from build123d import *

# Parameters (mm, degrees)
MODEL_R         = 0.65
MODEL_R_2       = 3.4746057
EXTRUDE_1_DEPTH = 0.5
EXTRUDE2_START  = -0.1
SKETCH2_R       = 0.65
SKETCH2_W       = 3.5
SKETCH2_H       = 2
EXTRUDE2_DEPTH  = 0.1
EXTRUDE1_START  = -0.5
EXTRUDE1_DEPTH  = 0.9


# Read off the part's stored shape, not the designer's step: Extrude1
with BuildPart() as part:
    # Model → Бобышка-Вытянуть1 (new, symmetric)
    with BuildSketch(Plane.XY):
        with BuildLine():
            Line((1024.38859, -762.8000398), (1024.38859, -762.0000398))
            Line((1024.38859, -762.0000398), (1012.53859, -762.0000398))
            Line((1012.53859, -762.0000398), (1012.53859, -773.0000398))
            Line((1012.53859, -773.0000398), (1024.38859, -773.0000398))
            Line((1024.38859, -773.0000398), (1024.38859, -772.2000398))
            ThreePointArc((1024.38859, -772.2000398), (1025.03859, -771.5500398), (1025.68859, -772.2000398))
            Line((1025.68859, -772.2000398), (1025.68859, -773.0000398))
            Line((1025.68859, -773.0000398), (1035.03859, -773.0000398))
            Line((1035.03859, -773.0000398), (1035.03859, -762.0000398))
            Line((1035.03859, -762.0000398), (1025.68859, -762.0000398))
            Line((1025.68859, -762.0000398), (1025.68859, -762.8000398))
            ThreePointArc((1025.68859, -762.8000398), (1025.03859, -763.4500398), (1024.38859, -762.8000398))
        make_face()
        with Locations((1033.53859, -767.5000398)):
            Circle(MODEL_R, mode=Mode.SUBTRACT)
        with Locations((1025.03859, -767.5000398)):
            Circle(MODEL_R_2, mode=Mode.SUBTRACT)
        with Locations((1014.03859, -767.5000398)):
            Circle(MODEL_R, mode=Mode.SUBTRACT)
    extrude(amount=EXTRUDE_1_DEPTH, both=True)

    # Sketch2 → Extrude2 (cut)
    # profile 1 of 2: a face of its own
    with BuildSketch(Plane.XY.offset(0.5).offset(EXTRUDE2_START)):
        Polygon((1020.33859, -764.0000398), (1020.33859, -762.0000398), (1012.53859, -762.0000398), (1012.53859, -773.0000398), (1020.33859, -773.0000398), (1020.33859, -771.0000398), (1020.33859, -769.0000398), (1020.33859, -766.0000398), align=None)
        with Locations((1014.03859, -767.5000398)):
            Circle(SKETCH2_R, mode=Mode.SUBTRACT)
        Polygon((1016.33859, -770.1000398), (1016.33859, -769.0000398), (1019.83859, -769.0000398), (1019.83859, -771.0000398), (1016.33859, -771.0000398), align=None, mode=Mode.SUBTRACT)
        with Locations((1018.08859, -767.5000398)):
            Rectangle(SKETCH2_W, SKETCH2_H, mode=Mode.SUBTRACT)
        Polygon((1019.83859, -764.0000398), (1019.83859, -766.0000398), (1016.33859, -766.0000398), (1016.33859, -764.9000398), (1016.33859, -764.0000398), align=None, mode=Mode.SUBTRACT)
    # profile 2 of 2: a face of its own
    with BuildSketch(Plane.XY.offset(0.5).offset(EXTRUDE2_START)):
        Polygon((1035.03859, -762.0000398), (1028.63859, -762.0000398), (1028.63859, -767.5000398), (1028.63859, -773.0000398), (1035.03859, -773.0000398), align=None)
        with Locations((1033.53859, -767.5000398)):
            Circle(SKETCH2_R, mode=Mode.SUBTRACT)
        Polygon((1029.13859, -769.1000398), (1029.13859, -767.5000398), (1029.13859, -765.9000398), (1032.13859, -765.9000398), (1032.13859, -767.5000398), (1032.13859, -769.1000398), align=None, mode=Mode.SUBTRACT)
    extrude(amount=EXTRUDE2_DEPTH, mode=Mode.SUBTRACT)

    # Extrude1 outline → Extrude1 (cut)
    with BuildSketch(Plane.XY.offset(EXTRUDE1_START)):
        with BuildLine():
            ThreePointArc((1013.81361784, -773.0000398), (1012.861518267, -770.322968067), (1012.53859, -767.5000398))
            Line((1012.53859, -767.5000398), (1012.53859, -773.0000398))
            Line((1012.53859, -773.0000398), (1013.81361784, -773.0000398))
        make_face()
        with BuildLine():
            ThreePointArc((1012.53859, -767.5000398), (1012.861518267, -764.677111533), (1013.81361784, -762.0000398))
            Line((1013.81361784, -762.0000398), (1012.53859, -762.0000398))
            Line((1012.53859, -762.0000398), (1012.53859, -767.5000398))
        make_face()
        with BuildLine():
            ThreePointArc((1033.390236544, -762.0000398), (1034.617641765, -764.629191967), (1035.03859, -767.5000398))
            Line((1035.03859, -767.5000398), (1035.03859, -762.0000398))
            Line((1035.03859, -762.0000398), (1033.390236544, -762.0000398))
        make_face()
        with BuildLine():
            ThreePointArc((1035.03859, -767.5000398), (1034.617641765, -770.370887633), (1033.390236544, -773.0000398))
            Line((1033.390236544, -773.0000398), (1035.03859, -773.0000398))
            Line((1035.03859, -773.0000398), (1035.03859, -767.5000398))
        make_face()
    extrude(amount=EXTRUDE1_DEPTH, mode=Mode.SUBTRACT)


solid = part.part
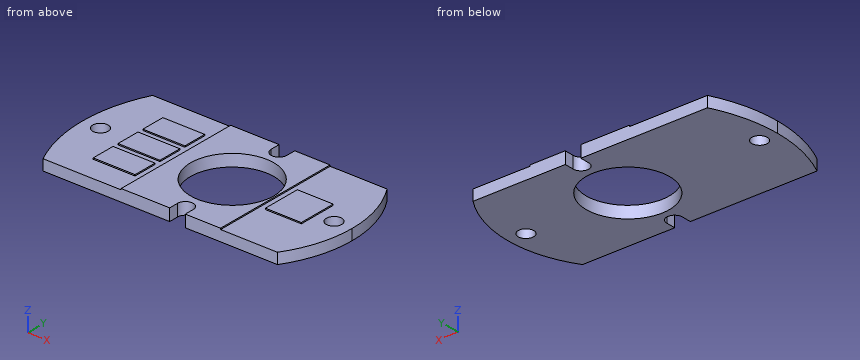
Model file for the job. Use its own axes, mm. Coordinates: 2 decimals unless noted, no trailing zeros. Write each loop counter-clockwise with the first axis right and the second up, starting at its lowest first coordinate (ties: lowest second). Pieces come first, ordered by that corner, then holes. Notation, with made-up numbers: (70, -11) -> (106, -11) arc R21 cw to (106, -2) -> close; hole circle Ø7 at (-32, 26.5). An arc over 180 degrees is marked (long way). One line per item, written item: value. Start each with the question number.
1) Flat gauge pin, fed straight in: pin 1 Ø0.6 at (y, z) = (-772.5, 0) entering from +X. Where does the tip first touch, or does it go through?
2) Slice it at B-B on y = -769.75. Write the cut outline in (x, z).
3) Slice it at C-C on x = 1024. Write the cut outline in (y, z).
4) Slice it at D-D on x = 1018.5. Write the cut outline in (y, z).
5) Slice it at A-A on z = 0.1. Write the cut outline in (x, y), then the cut area to 3 significant figures.
6) Probe probe 1 along X at (y, z) = (-767.5, -0.2); probe 2 along Y at (x, z) = (1025, 0.35); probe 3 along Y at (x, z) = (1014, 0.15). List the from-to ranges inside material, lowest first.
Answers follow:
1. pin 1: x = 1033.87
2. outline: (1012.74, -0.5) -> (1022.39, -0.5) -> (1022.39, 0.5) -> (1020.34, 0.5) -> (1020.34, 0.4) -> (1019.84, 0.4) -> (1019.84, 0.5) -> (1016.34, 0.5) -> (1016.34, 0.4) -> (1012.74, 0.4) -> close; (1027.69, -0.5) -> (1034.78, -0.5) -> (1034.78, 0.4) -> (1028.64, 0.4) -> (1028.64, 0.5) -> (1027.69, 0.5) -> close
3. outline: (-773, -0.5) -> (-770.82, -0.5) -> (-770.82, 0.5) -> (-773, 0.5) -> close; (-764.18, -0.5) -> (-762, -0.5) -> (-762, 0.5) -> (-764.18, 0.5) -> close
4. outline: (-773, -0.5) -> (-762, -0.5) -> (-762, 0.4) -> (-764, 0.4) -> (-764, 0.5) -> (-766, 0.5) -> (-766, 0.4) -> (-766.5, 0.4) -> (-766.5, 0.5) -> (-768.5, 0.5) -> (-768.5, 0.4) -> (-769, 0.4) -> (-769, 0.5) -> (-771, 0.5) -> (-771, 0.4) -> (-773, 0.4) -> close
5. outline: (1013.81, -773) -> (1024.39, -773) -> (1024.39, -772.2) arc R0.65 cw to (1025.69, -772.2) -> (1025.69, -773) -> (1033.39, -773) arc R10 ccw to (1033.39, -762) -> (1025.69, -762) -> (1025.69, -762.8) arc R0.65 cw to (1024.39, -762.8) -> (1024.39, -762) -> (1013.81, -762) arc R12.5 ccw to start; hole circle Ø1.3 at (1014.04, -767.5); hole circle Ø6.95 at (1025.04, -767.5); hole circle Ø1.3 at (1033.54, -767.5)
5. area: 193 mm2
6. probe 1: 1012.54 to 1013.39, 1014.69 to 1021.56, 1028.51 to 1032.89, 1034.19 to 1035.04
6. probe 2: -771.55 to -770.97, -764.03 to -763.45
6. probe 3: -773 to -768.15, -766.85 to -762
